from build123d import *

# Parameters (mm, degrees)
BOSS_EXTRUDE1_DEPTH            = 6.35
BOSS_EXTRUDE2_DEPTH            = 3.175
BOSS_EXTRUDE3_DEPTH            = 3.175
CUT_EXTRUDE1_DEPTH             = 3.175
SKETCH5_W                      = 5.08
SKETCH5_H                      = 13.208
CUT_EXTRUDE2_DEPTH             = 7.35
SKETCH6_W                      = 5.08
SKETCH6_H                      = 13.208
CUT_EXTRUDE3_DEPTH             = 7.35
CUT_EXTRUDE4_REACH             = 60.039
CUT_EXTRUDE5_DEPTH             = 3.175
CUT_EXTRUDE6_DEPTH             = 7.35
CUT_EXTRUDE7_DEPTH             = 7.35
CUT_EXTRUDE8_DEPTH             = 7.35
CUT_EXTRUDE9_DEPTH             = 10.525
CUT_EXTRUDE10_DEPTH            = 2.032
F_12_CLEARANCE_HOLE1_D         = 6.096
F_12_CLEARANCE_HOLE1_DEPTH     = 4.953
F_3_CLEARANCE_HOLE1_D          = 2.921
F_3_CLEARANCE_HOLE1_DEPTH      = 9.525
F_7_0_201_DIAMETER_HOLE1_D     = 5.1054
F_7_0_201_DIAMETER_HOLE1_DEPTH = 9.525
FILLET1_R                      = 3.175
FILLET2_R                      = 0.8255
FILLET3_R                      = 1
FILLET4_R                      = 6.35


with BuildPart() as part:
    # Sketch1 → Boss-Extrude1 (new body)
    with BuildSketch(Plane(origin=(0, 0, 0), x_dir=(-1, 0, 0), z_dir=(0, 0, -1))):
        Polygon((-50.8, 863.6), (-66.04, 857.25), (-66.04, 844.55), (-50.8, 838.2), (0, 838.2), (15.24, 844.55), (15.24, 857.25), (0, 863.6), align=None)
    extrude(amount=-BOSS_EXTRUDE1_DEPTH)

    # Sketch2 → Boss-Extrude2 (add)
    with BuildSketch(Plane(origin=(0, 0, 0), x_dir=(-1, 0, 0), z_dir=(0, 0, -1))):
        Polygon((-50.8762, 838.23175), (-66.04, 844.55), (-66.04, 857.25), (-50.8762, 863.56825), align=None)
    extrude(amount=BOSS_EXTRUDE2_DEPTH)

    # Sketch3 → Boss-Extrude3 (add)
    with BuildSketch(Plane(origin=(0, 0, 0), x_dir=(-1, 0, 0), z_dir=(0, 0, -1))):
        Polygon((0.0762, 863.56825), (15.24, 857.25), (15.24, 844.55), (0.0762, 838.23175), align=None)
    extrude(amount=BOSS_EXTRUDE3_DEPTH)

    # Sketch4 → Cut-Extrude1 (cut)
    with BuildSketch(Plane(origin=(0, 0, -3.175), x_dir=(-1, 0, 0), z_dir=(0, 0, -1))):
        Polygon((2.286, 862.6475), (2.286, 839.1525), (15.24, 844.55), (15.24, 857.25), align=None)
    extrude(amount=-CUT_EXTRUDE1_DEPTH, mode=Mode.SUBTRACT)

    # Sketch5 → Cut-Extrude2 (cut, through all)
    with BuildSketch(Plane(origin=(0, 0, 0), x_dir=(-1, 0, 0), z_dir=(0, 0, -1))):
        with Locations((-5.461, 850.9)):
            Rectangle(SKETCH5_W, SKETCH5_H)
    extrude(amount=-CUT_EXTRUDE2_DEPTH, mode=Mode.SUBTRACT)

    # Sketch6 → Cut-Extrude3 (cut, through all)
    with BuildSketch(Plane(origin=(0, 0, 0), x_dir=(-1, 0, 0), z_dir=(0, 0, -1))):
        with Locations((-45.339, 850.9)):
            Rectangle(SKETCH6_W, SKETCH6_H)
    extrude(amount=-CUT_EXTRUDE3_DEPTH, mode=Mode.SUBTRACT)

    # Sketch7 → Cut-Extrude4 (cut, up to next)
    with BuildSketch(Plane.ZY.offset(-8.001), mode=Mode.PRIVATE) as cut_extrude4_sk1:
        with BuildLine():
            Line((6.35, 847.702120834), (6.35, 854.097879166))
            ThreePointArc((6.35, 854.097879166), (3.2766, 850.9), (6.35, 847.702120834))
        make_face()
    cut_extrude4_tool1 = extrude(cut_extrude4_sk1.sketch, amount=-CUT_EXTRUDE4_REACH, mode=Mode.PRIVATE) & part.part
    add(cut_extrude4_tool1.solids().sort_by_distance((8.001, 850.9, 5.049826))[0], mode=Mode.SUBTRACT)

    # Sketch8 → Cut-Extrude5 (cut)
    with BuildSketch(Plane(origin=(0, 0, -3.175), x_dir=(-1, 0, 0), z_dir=(0, 0, -1))):
        Polygon((-53.086, 839.1525), (-53.086, 862.6475), (-66.04, 857.25), (-66.04, 844.55), align=None)
    extrude(amount=-CUT_EXTRUDE5_DEPTH, mode=Mode.SUBTRACT)

    # Sketch9 → Cut-Extrude6 (cut, through all)
    with BuildSketch(Plane(origin=(0, 0, 0), x_dir=(-1, 0, 0), z_dir=(0, 0, -1))):
        with BuildLine():
            Line((-35.56, 840.1558), (-32.340549132, 840.1558))
            ThreePointArc((-32.340549132, 840.1558), (-29.851349132, 842.645), (-32.340549132, 845.1342))
            Line((-32.340549132, 845.1342), (-35.56, 845.1342))
            ThreePointArc((-35.56, 845.1342), (-38.0492, 842.645), (-35.56, 840.1558))
        make_face()
    extrude(amount=-CUT_EXTRUDE6_DEPTH, mode=Mode.SUBTRACT)

    # Sketch10 → Cut-Extrude7 (cut, through all)
    with BuildSketch(Plane(origin=(0, 0, 0), x_dir=(-1, 0, 0), z_dir=(0, 0, -1))):
        with BuildLine():
            Line((-35.56, 861.6442), (-38.1508, 861.6442))
            ThreePointArc((-38.1508, 861.6442), (-40.64, 859.155), (-38.1508, 856.6658))
            Line((-38.1508, 856.6658), (-35.56, 856.6658))
            ThreePointArc((-35.56, 856.6658), (-33.0708, 859.155), (-35.56, 861.6442))
        make_face()
    extrude(amount=-CUT_EXTRUDE7_DEPTH, mode=Mode.SUBTRACT)

    # Sketch11 → Cut-Extrude8 (cut, through all)
    with BuildSketch(Plane(origin=(0, 0, 0), x_dir=(-1, 0, 0), z_dir=(0, 0, -1))):
        with BuildLine():
            Line((-15.24, 845.1342), (-18.4658, 845.1342))
            ThreePointArc((-18.4658, 845.1342), (-20.955, 842.645), (-18.4658, 840.1558))
            Line((-18.4658, 840.1558), (-15.24, 840.1558))
            ThreePointArc((-15.24, 840.1558), (-12.7508, 842.645), (-15.24, 845.1342))
        make_face()
    extrude(amount=-CUT_EXTRUDE8_DEPTH, mode=Mode.SUBTRACT)

    # Sketch12 → Cut-Extrude9 (cut, through all)
    with BuildSketch(Plane.XY.offset(6.35)):
        with BuildLine():
            Line((15.24, 861.6442), (12.6492, 861.6442))
            ThreePointArc((12.6492, 861.6442), (10.16, 859.155), (12.6492, 856.6658))
            Line((12.6492, 856.6658), (15.24, 856.6658))
            ThreePointArc((15.24, 856.6658), (17.7292, 859.155), (15.24, 861.6442))
        make_face()
    extrude(amount=-CUT_EXTRUDE9_DEPTH, mode=Mode.SUBTRACT)

    # Sketch13 → Cut-Extrude10 (cut)
    with BuildSketch(Plane(origin=(0, 0, 0), x_dir=(-1, 0, 0), z_dir=(0, 0, -1))):
        with BuildLine():
            Line((-26.8605, 843.0006), (-23.940383746, 843.0006))
            Line((-23.940383746, 843.0006), (-23.940383746, 858.7994))
            ThreePointArc((-23.940383746, 858.7994), (-25.374596157, 860.310479047), (-26.8605, 858.8502))
            Line((-26.8605, 858.8502), (-26.8605, 843.0006))
        make_face()
    extrude(amount=-CUT_EXTRUDE10_DEPTH, mode=Mode.SUBTRACT)

    # #12 Clearance Hole1
    with Locations(Plane.XY.offset(6.35)):
        with Locations((25.4, 858.8502)):
            Hole(F_12_CLEARANCE_HOLE1_D / 2, depth=F_12_CLEARANCE_HOLE1_DEPTH)

    # #3 Clearance Hole1
    with Locations(Plane.XY.offset(6.35)):
        with Locations((25.4, 842.9498)):
            Hole(F_3_CLEARANCE_HOLE1_D / 2, depth=F_3_CLEARANCE_HOLE1_DEPTH)

    # #7 (0.201) Diameter Hole1
    with Locations(Plane.XY.offset(6.35)):
        with Locations((-9.525, 850.9), (60.325, 850.9)):
            Hole(F_7_0_201_DIAMETER_HOLE1_D / 2, depth=F_7_0_201_DIAMETER_HOLE1_DEPTH)

    # Fillet1
    fillet1_edges = [part.edges().sort_by_distance(p)[0] for p in [
        (0, 838.2, 3.175),
        (50.8, 838.2, 3.175),
        (50.8, 863.6, 3.175),
        (0, 863.6, 3.175),
    ]]
    fillet(fillet1_edges, radius=FILLET1_R)

    # Fillet2
    fillet2_edges = [part.edges().sort_by_distance(p)[0] for p in [
        (8.001, 857.504, 3.175),
        (2.921, 857.504, 3.175),
        (2.921, 844.296, 3.175),
        (8.001, 844.296, 3.175),
        (47.879, 857.504, 3.175),
        (42.799, 857.504, 3.175),
        (42.799, 844.296, 3.175),
        (47.879, 844.296, 3.175),
    ]]
    fillet(fillet2_edges, radius=FILLET2_R)

    # Fillet3
    fillet3_edges = [part.edges().sort_by_distance(p)[0] for p in [
        (52.236076923, 838.798365385, -3.175),
        (-1.436076923, 838.798365385, -3.175),
        (-0.334631427, 863.448316043, -3.175),
        (-0.334631427, 838.351683957, -3.175),
        (52.236076923, 863.001634615, -3.175),
        (51.134631427, 863.448316043, -3.175),
        (51.134631427, 838.351683957, -3.175),
        (-1.436076923, 863.001634615, -3.175),
    ]]
    fillet(fillet3_edges, radius=FILLET3_R)

    # Fillet4
    fillet4_edges = [part.edges().sort_by_distance(p)[0] for p in [
        (-15.24, 857.25, 3.175),
        (-15.24, 844.55, 3.175),
        (66.04, 844.55, 3.175),
        (66.04, 857.25, 3.175),
    ]]
    fillet(fillet4_edges, radius=FILLET4_R)


solid = part.part
Here's how the part is built. I have some questions about the finished solid (model axes, mm). A direction names the side the tool comes from. Give positions to 0.01 mm unless a question says otherwise; leave off trailing zeros. Order: outer loops, then holes, each group sorted by start corner. A loop starts at its lowest first (then second) coordinate and runs counter-clockwise, first axis right, second up. Notation, with made-up numbers: (-9, -0.75) -> (17, -0.75) arc R20 ccw to (17, 8.25) -> close; hole circle Ø1 at (83, 54). An arc over 180 degrees is marked (long way). One line per item, written item: value. Start each with the question number.
1. For faces 1 (the face through (31, 851, 0)), 2 (the face through (45, 857.504, 3)), 3 (the face through (-2.286, 851, -2)), which set-ups out of +Z, -Z, +X, -X, +Y, -Y let a thin tool reach every point of the face, with its end or its side?
2. I need wall thicknesses on probe 1 along X at (y, z) = (850.9, 4.5); probe 2 along X at (y, z) = (850.9, 1.5); probe 3 along Y at (x, z) = (25.4, 4.55). Which ranges of each line are inside material? Lowest first, please. Write a range as from..to.
3. Will these pins go through, and if not, where does the flat tip stop? pin 1 Ø5 at (y, z) = (857, 2) entering from +X; pin 2 Ø3.5 at (y, z) = (851.5, -2) entering from +X; pin 3 Ø3 at (y, z) = (859.5, 0) entering from -X.
4. Imagine slicing it at B-B, the plane y = 850.9. Count the separate pieces of the cut face and the enclosed holes in it, plus the area to 3 significant figures.
5. Imagine slicing it at A-A, the plane x = 25.4. List the corners of the cut face in (y, z) for me, plus the area to 3 significant figures.
6. We'd pull the mould along X, two halves only. Please class faces 4 (the face through (5, 857.504, 3)), 5 (the face through (26, 838.2, 3)), 6 (the face through (-1.504, 839.136, -2.874)): released by +X, released by -X, zero draft, split by the parting line, or undercut.
7. Imagine slicing it at C-C, the plane x = -8.5. List the corners of the cut face in (y, z) for me.
Values follow:
1. face 1: -Z, +Y, -Y
1. face 2: +Z, -Z
1. face 3: -Z, -X, +Y, -Y
2. probe 1: x = -15.24..-12.08, -6.97..2.92, 47.88..57.77, 62.88..66.04
2. probe 2: x = -15.24..-12.08, -6.97..2.92, 8..23.94, 26.86..42.8, 47.88..57.77, 62.88..66.04
2. probe 3: y = 838.2..841.49, 844.41..848.34, 853.46..855.8, 861.9..863.6
3. pin 1: stops at x = 65.86
3. pin 2: stops at x = 53.09
3. pin 3: stops at x = -12.83
4. separate pieces: 5
4. enclosed holes: 0
4. area: 288 mm2
5. outline: (838.2, 0) -> (841.49, 0) -> (841.49, 6.35) -> (838.2, 6.35) -> close; (844.41, 2.03) -> (855.8, 2.03) -> (855.8, 6.35) -> (854.1, 6.35) arc R3.2 cw to (847.7, 6.35) -> (844.41, 6.35) -> close; (860.31, 0) -> (863.6, 0) -> (863.6, 6.35) -> (861.9, 6.35) -> (861.9, 1.4) -> (860.31, 1.4) -> close
5. area: 67.8 mm2
6. face 4: undercut
6. face 5: zero draft
6. face 6: released by -X
7. outline: (841.74, 0) -> (848.56, 0) -> (848.56, 6.35) -> (841.74, 6.35) -> close; (853.24, 0) -> (860.06, 0) -> (860.06, 6.35) -> (853.24, 6.35) -> close
